Verification items for the finished model (mm, model axes). Face numbers are marked on the shaded views. A direction names the side the tool comes from. Coordinates: 2 decimals unless noted, no trailing zeros. Order: outer loops, then holes, each group sorted by start corner. A loop starts at its lowest first (then second) coordinate and runs counter-clockwise, first axis right, second up. Notation, with made-up numbers: (16.25, 66.25) -> (32.25, 66.25) arc R22 ccw to (32.25, 74.25) -> close; hole circle Ø2 at (33, 78.5). An arc over 180 degrees is marked (long way). Write item = value, one per line. Start each with the question number.
1. Cross-section at A-A on z = 48. Record the cut outline in (x, y), plus the area to 3 significant figures.
2. Cross-section at D-D on x = 116. Record the cut outline in (y, z).
3. Thickness scan on line 1 along Z through (x, y) = (88.5, -97); line 2 along X through (y, z) = (-39, 46.5); line 3 along X through (y, z) = (-48, 13.5). Record the ranges inside material, lowest first. Write a range as from..to.
4. Set-up check for the marked faces 1 and 2: record each of +Z, -Z, +X, -X, +Y, -Y from which the full face is reachable in a straight line by a thin tool's end or side.
5. Go/stop test with flat-tipped pins: P1, Ø12, axis at x = 50, z = 45.5, coming from the +Y side (3 decimals); P2, Ø10, axis at x = 101.5, z = 34.5, coming from the -Y side; P3, Ø3, axis at y = -79.5, z = 36.5, coming from the -X side. Record where each tip stops, or that it passes through.
6. Cross-section at C-C on y = -98.5. Record the cut outline in (x, z), plus the area to 3 significant figures.
7. Cross-section at B-B on x = 81.5. Record the cut outline in (y, z), plus the area to 3 significant figures.
from build123d import *

# Parameters (mm, degrees)
F0_W     = 152.4
F0_H     = 114.3
F1_DEPTH = 12.7
F3_DEPTH = 38.1


with BuildPart() as f1:
    # F0 (on Top) → F1 (new body)
    with BuildSketch(Plane.XY):
        with Locations((76.2, -57.15)):
            Rectangle(F0_W, F0_H)
    extrude(amount=F1_DEPTH)

    # F2 (on face) → F3 (join)
    with BuildSketch(Plane.XY.offset(12.7)):
        Polygon((76.2, -41.275), (55.0333333333, -57.15), (76.2, -57.15), align=None)
        with BuildLine():
            Line((76.2, -57.15), (55.0333333333, -57.15))
            Line((55.0333333333, -57.15), (46.228, -63.754))
            ThreePointArc((46.228, -63.754), (55.6440512242, -61.3416414305), (64.008, -66.294))
            Line((64.008, -66.294), (76.2, -57.15))
        make_face()
        with BuildLine():
            Line((88.392, -48.006), (76.2, -57.15))
            Line((76.2, -57.15), (97.3666666667, -57.15))
            Line((97.3666666667, -57.15), (106.172, -50.546))
            ThreePointArc((106.172, -50.546), (96.7559487758, -52.9583585695), (88.392, -48.006))
        make_face()
        Polygon((97.3666666667, -57.15), (76.2, -57.15), (76.2, -73.025), align=None)
        with BuildLine():
            Line((76.2, -41.275), (76.2, -57.15))
            Line((76.2, -57.15), (88.392, -48.006))
            ThreePointArc((88.392, -48.006), (85.9796414305, -38.5899487758), (90.932, -30.226))
            Line((90.932, -30.226), (76.2, -41.275))
        make_face()
        with BuildLine():
            Line((76.2, -73.025), (76.2, -57.15))
            Line((76.2, -57.15), (64.008, -66.294))
            ThreePointArc((64.008, -66.294), (65.8962778852, -69.8979073716), (66.548, -73.914))
            ThreePointArc((66.548, -73.914), (65.2072253257, -79.5936126628), (61.468, -84.074))
            Line((61.468, -84.074), (76.2, -73.025))
        make_face()
        with BuildLine():
            ThreePointArc((64.008, -66.294), (55.6440512242, -61.3416414305), (46.228, -63.754))
            Line((46.228, -63.754), (53.848, -73.914))
            Line((53.848, -73.914), (64.008, -66.294))
        make_face()
        with BuildLine():
            Line((53.848, -73.914), (46.228, -63.754))
            ThreePointArc((46.228, -63.754), (41.2756414305, -72.1179487758), (43.688, -81.534))
            Line((43.688, -81.534), (53.848, -73.914))
        make_face()
        with BuildLine():
            ThreePointArc((90.932, -30.226), (85.9796414305, -38.5899487758), (88.392, -48.006))
            Line((88.392, -48.006), (98.552, -40.386))
            Line((98.552, -40.386), (90.932, -30.226))
        make_face()
        with BuildLine():
            Line((98.552, -40.386), (88.392, -48.006))
            ThreePointArc((88.392, -48.006), (96.7559487758, -52.9583585695), (106.172, -50.546))
            Line((106.172, -50.546), (98.552, -40.386))
        make_face()
        with BuildLine():
            ThreePointArc((66.548, -73.914), (65.8962778852, -69.8979073716), (64.008, -66.294))
            Line((64.008, -66.294), (53.848, -73.914))
            Line((53.848, -73.914), (61.468, -84.074))
            ThreePointArc((61.468, -84.074), (65.2072253257, -79.5936126628), (66.548, -73.914))
        make_face()
        with BuildLine():
            ThreePointArc((108.712, -32.766), (100.3480512242, -27.8136414305), (90.932, -30.226))
            Line((90.932, -30.226), (98.552, -40.386))
            Line((98.552, -40.386), (108.712, -32.766))
        make_face()
        with BuildLine():
            Line((61.468, -84.074), (53.848, -73.914))
            Line((53.848, -73.914), (43.688, -81.534))
            ThreePointArc((43.688, -81.534), (52.0519487758, -86.4863585695), (61.468, -84.074))
        make_face()
        with BuildLine():
            Line((98.552, -40.386), (106.172, -50.546))
            ThreePointArc((106.172, -50.546), (109.9112253257, -46.0656126628), (111.252, -40.386))
            ThreePointArc((111.252, -40.386), (110.6002778852, -36.3699073716), (108.712, -32.766))
            Line((108.712, -32.766), (98.552, -40.386))
        make_face()
    extrude(amount=F3_DEPTH)


solid = f1.part
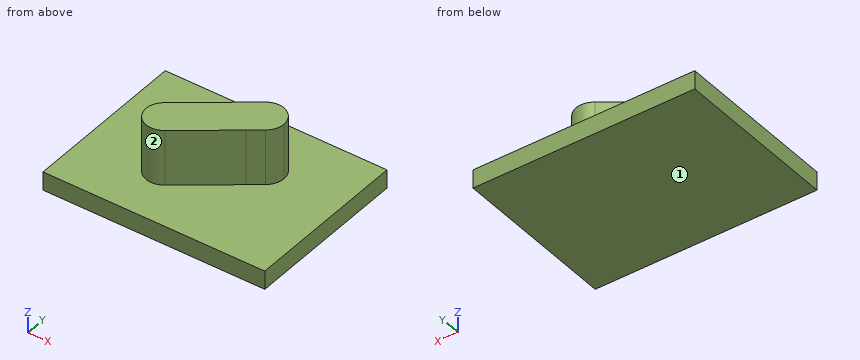
Worked out:
q1.outline = (46.23, -63.75) arc R12.7 ccw to (61.47, -84.07) -> (106.17, -50.55) arc R12.7 ccw to (90.93, -30.23) -> close
q1.area = 1,930 mm²
q2.outline = (-114.3, 0) -> (0, 0) -> (0, 12.7) -> (-114.3, 12.7) -> close
q3.line_1 = 0..12.7
q3.line_2 = 79.23..111.18
q3.line_3 = 67.23..108.72
q4.face_1 = -Z, +X, -X, +Y, -Y
q4.face_2 = +Z
q5.P1 = -56.425
q5.P2 = -57.8
q5.P3 = 41.82
q6.outline = (0, 0) -> (152.4, 0) -> (152.4, 12.7) -> (0, 12.7) -> close
q6.area = 1,940 mm²
q7.outline = (-114.3, 0) -> (0, 0) -> (0, 12.7) -> (-37.3, 12.7) -> (-37.3, 50.8) -> (-69.05, 50.8) -> (-69.05, 12.7) -> (-114.3, 12.7) -> close
q7.area = 2,660 mm²
